Build history of the part. All positions in model axes, mm. A direction names the side the tool comes from. Round coordinates to 2 decimals unless told otherwise and drop trailing zeros. Write each loop counter-clockwise with the first axis right and the second up, starting at its lowest first coordinate (ties: lowest second). Pieces come first, ordered by that corner, then holes. Notation, with made-up numbers: (38, 6.25) - (43, 6.25) arc R32 cw to (43, 40.25) - close; hole circle Ø4 at (-21.5, 5.25). An arc over 180 degrees is marked (long way). Write each question's results on one line, items separated by ' | '.
Autodesk Inventor part; units mm, degrees
ref_plane "YZ Plane" through (0, 0, 0) normal (1, 0, 0) x (0, 1, 0)
ref_plane "XZ Plane" through (0, 0, 0) normal (0, 1, 0) x (-1, 0, 0)
ref_plane "XY Plane" through (0, 0, 0) normal (0, 0, 1) x (1, 0, 0)
sketch "Sketch1" plane through (0, 0, 0) normal (0, 0, 1) x (1, 0, 0)
  circle A0 centre (0, 0) radius 20
  dimension "d0" = 40
extrude "Extrusion1" add sketch "Sketch1" along normal mid plane 3
sketch "Sketch2" plane through (0, 0, 1.5) normal (0, 0, 1) x (1, 0, 0)
  circle A0 centre (0, 0) radius 15
  dimension "d3" = 30
extrude "Extrusion2" add sketch "Sketch2" along normal blind 1.5
sketch "Sketch3" plane through (0, 0, -1.5) normal (0, 0, -1) x (-1, 0, 0)
  circle A0 centre (0, 0) radius 17.5 construction
  point P0 (0, 17.5)
  dimension "d6" = 35
hole "Hole1" at (0, 17.5, -1.5) direction (0, 0, 1) diameter 3 depth 3
pattern_circular "Circular Pattern1" count 6 over 360 about axis through (0, 0, 0) along (0, 0, 1) of "Hole1"
sketch "Sketch4" plane through (0, 0, -1.5) normal (0, 0, -1) x (-1, 0, 0)
  circle A0 centre (0, 0) radius 6
  dimension "d17" = 12
extrude "Extrusion3" add sketch "Sketch4" along normal blind 6
thread "Thread1"
sketch "Sketch8" plane through (0, 0, -7.5) normal (0, 0, -1) x (-1, 0, 0)
  circle A0 centre (0, 0) radius 6
hole "Hole5" at (0, 0, -7.5) direction (0, 0, 1) diameter 6 depth 10.5 countersink diameter 7 countersink angle 90
properties part number "14"
(1) Drill centre lines: probe 1 along Y at (x, z) = (15, 1.25); probe 2 along Y at (x, z) = (16, -1.25); probe 3 along X at (y, z) = (8.75, 0.85). Where is each one in solid material? Low to high. Write a range as [from, to].
Worked answers:
probe 1: y = [-13.23, -10.24], [-7.26, 7.26], [10.24, 13.23] | probe 2: y = [-12, -9.99], [-7.51, 7.51], [9.99, 12] | probe 3: x = [-17.98, -16.66], [-13.66, 13.66], [16.66, 17.98]
(2) Slice it at A-A, the plane x = 0. Write the cut outline in (y, z).
Worked answers:
outline: (-20, -1.5) - (-19, -1.5) - (-19, 1.5) - (-20, 1.5) - close; (-16, -1.5) - (-6, -1.5) - (-6, -7.5) - (-3.5, -7.5) - (-3, -7) - (-3, 3) - (-15, 3) - (-15, 1.5) - (-16, 1.5) - close; (3, -7) - (3.5, -7.5) - (6, -7.5) - (6, -1.5) - (16, -1.5) - (16, 1.5) - (15, 1.5) - (15, 3) - (3, 3) - close; (19, -1.5) - (20, -1.5) - (20, 1.5) - (19, 1.5) - close
(3) Flat gauge pins, fed straight in: pin 1 Ø3 at (y, z) = (3.5, -1.5) entering from +X; pin 2 Ø6 at (y, z) = (-12.5, -2) entering from -X; pin 3 Ø1.8 at (x, y) = (15.16, -8.75) entering from -Z; pin 4 Ø5 at (x, y) = (-14.5, 11) entering from -Z. Where does each tip first touch, or does it go through?
Worked answers:
pin 1: stops at x = 19.9 | pin 2: stops at x = -17.58 | pin 3: passes through | pin 4: stops at z = -1.5
(4) Two-plate mould, pull along Y, no slides. Class faces 1 (the cylindrical face through (-14.985, -0.66, 2.24)), 2 (the flat face through (4, 5, -1.5)), 3 (the cylindrical face through (16.643, 8.945, 0.021)), 4 (the cylindrical face through (0, -3, -2)): released by +Y, released by -Y, zero draft, split by the parting line, or undercut.
Worked answers:
face 1: split by the parting line | face 2: zero draft | face 3: undercut | face 4: undercut
(5) Tool access for faces 5 (the cylindrical face through (6, 0, -4)), 6 (the flat face through (3, 15, 1.5)), 7 (the cylindrical face through (16.62, -9.08, 0.02)): list every direction of +Z, -Z, +X, -X, +Y, -Y with a clear straight run to the whole face (end or side of a thin tool).
Worked answers:
face 5: -Z | face 6: +Z | face 7: +Z, -Z
(6) Slice it at D-D, the plane z = -6.5. Write the cut outline in (x, y), and give its area (3 significant figures).
Worked answers:
outline: circle Ø12 at (0, 0); hole circle Ø6 at (0, 0) | area: 84.8 mm2
(7) Slice it at B-B, the plane y = 0. Write the cut outline in (x, z).
Worked answers:
outline: (-20, -1.5) - (-6, -1.5) - (-6, -7.5) - (-3.5, -7.5) - (-3, -7) - (-3, 3) - (-15, 3) - (-15, 1.5) - (-20, 1.5) - close; (3, -7) - (3.5, -7.5) - (6, -7.5) - (6, -1.5) - (20, -1.5) - (20, 1.5) - (15, 1.5) - (15, 3) - (3, 3) - close
(8) Slice it at C-C, the plane z = 1. Write the cut outline in (x, y), and give its area (3 significant figures).
Worked answers:
outline: circle Ø40 at (0, 0); hole circle Ø3 at (-15.16, -8.75); hole circle Ø3 at (-15.16, 8.75); hole circle Ø6 at (0, 0); hole circle Ø3 at (0, -17.5); hole circle Ø3 at (0, 17.5); hole circle Ø3 at (15.16, -8.75); hole circle Ø3 at (15.16, 8.75) | area: 1,190 mm2
